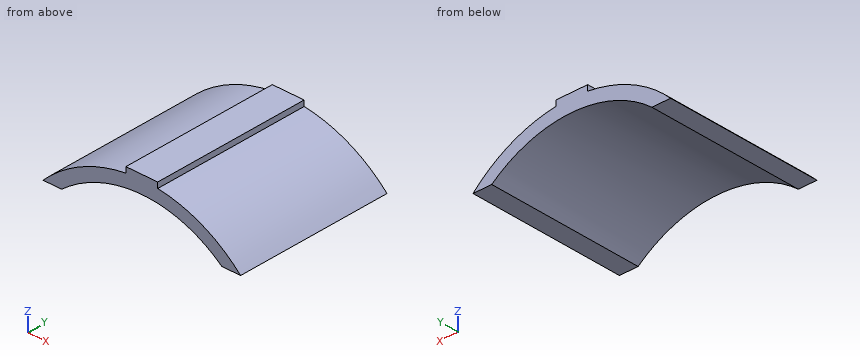
from build123d import *

# Parameters (mm, degrees)
BOSS_EXTRUDE1_DEPTH = 25


with BuildPart() as part:
    # Sketch1 → Boss-Extrude1 (new body)
    with BuildSketch(Plane(origin=(0, 0, 0), x_dir=(1, 0, 0), z_dir=(0, 1, 0))):
        with BuildLine():
            Line((-15.653135277, -15.458957145), (-12.689391002, -15.458957145))
            ThreePointArc((-12.689391002, -15.458957145), (0, -20), (12.689391002, -15.458957145))
            Line((12.689391002, -15.458957145), (15.653135277, -15.458957145))
            ThreePointArc((15.653135277, -15.458957145), (9.634106681, -19.778371734), (2.522561476, -21.854900677))
            Line((2.522561476, -21.854900677), (2.522561476, -22.740089193))
            Line((2.522561476, -22.740089193), (-2.522561476, -22.740089193))
            Line((-2.522561476, -22.740089193), (-2.522561476, -21.854900677))
            ThreePointArc((-2.522561476, -21.854900677), (-9.634106681, -19.778371734), (-15.653135277, -15.458957145))
        make_face()
    extrude(amount=BOSS_EXTRUDE1_DEPTH)


solid = part.part
CAD build for the part. Positions are in the model's coordinates, mm. Round coordinates to 2 decimals unless told otherwise and drop trailing zeros. Order: outer loops, then holes, each group sorted by start corner. A loop starts at its lowest first (then second) coordinate and runs counter-clockwise, first axis right, second up. Notation, with made-up numbers: M 6.25,27 L 15.25,27 A34 cw 15.25,58 Z; hole C 63,2 d4. An arc over 180 degrees is marked long. Use one line per item in the form item = value.
Q1. Saw through at C-C on z = 17. Give the cut face in (x, y).
Recorded:
outline = M -13.96,0 L -10.54,0 L -10.54,25 L -13.96,25 Z; M 10.54,0 L 13.96,0 L 13.96,25 L 10.54,25 Z
Q2. Saw through at B-B on z = 19.5. Give the cut face in (x, y), then the cut area to 3 significant figures.
Recorded:
outline = M -10.19,0 L -4.44,0 L -4.44,25 L -10.19,25 Z; M 4.44,0 L 10.19,0 L 10.19,25 L 4.44,25 Z
area = 287 mm^2
Q3. Probe L1, parallel to X at y = 6.5, z = 18; L2, parallel to X at y = 6, z = 16; L3, parallel to X at y = 2.25, z = 22.5. List the from-to ranges inside material, lowest first.
Recorded:
L1 = -12.65 to -8.72, 8.72 to 12.65
L2 = -15.1 to -12, 12 to 15.1
L3 = -2.52 to 2.52
Q4. Saw through at D-D on x = 4.5. Give the cut face in (y, z), then the cut area to 3 significant figures.
Recorded:
outline = M 0,19.49 L 25,19.49 L 25,21.53 L 0,21.53 Z
area = 51.2 mm^2
Q5. Saw through at A-A on y = 16. Give the cut face in (x, z).
Recorded:
outline = M -15.65,15.46 L -12.69,15.46 A20 cw 12.69,15.46 L 15.65,15.46 A22 ccw 2.52,21.85 L 2.52,22.74 L -2.52,22.74 L -2.52,21.85 A22 ccw Z
Q6. Flat gauge pins, fed straight in: P1, Ø4, axis at y = 7.5, z = 18, coming from the +X side; P2, Ø6, axis at x = 8.5, y = 15, coming from the +Z side. Where does each tip first touch, or does it go through?
Recorded:
P1 = 15.1
P2 = 21.3
